Verification items for the finished model (mm, model axes). A direction names the side the tool comes from. Give positions to 0.01 mm unless a question says otherwise; leave off trailing zeros. Write each loop counter-clockwise with the first axis right and the second up, starting at its lowest first coordinate (ties: lowest second). Pieces come first, ordered by that corner, then holes. Notation, with made-up numbers: (-17, 13) -> (37, 13) arc R24 ccw to (37, 50) -> close; hole circle Ø1 at (20, 13.25). An arc over 180 degrees is marked (long way). Answer as CSV lines item,"result". Start each with the question number.
1) Sectioned sample at D-D on z = 0. Record the cut outline in (x, y).
2) Material ranges on L1, parallel to X at y = 4.25, z = -4.5; L2, parallel to Y at x = 0.5, z = -6.25; L3, parallel to X at y = 8.5, z = 0, recorded low to high.
3) Sectioned sample at B-B on z = -7. Record the cut outline in (x, y).
4) Sectioned sample at C-C on y = 11.5. Record the cut outline in (x, z).
5) Sectioned sample at A-A on x = 6. Record the cut outline in (y, z).
6) Tool access check on faces 1 (the flat face through (10, 6, 6)), 2 (the cylindrical face through (13.468, 14.409, 0.759)), 3 (the flat face through (-7, 8, -3)), 4 (the flat face through (4, 6, 0)), 5 (the flat face through (10, 6, -6)). Record the directions out of +Z, -Z, +X, -X, +Y, -Y that give a thin tool (end or side, any length) a straight path to the whole face; none if there is none.
7) Mould release check, pull along X, two halves, no side actions. Record for faces 6 (the flat face through (-11, 8, -6)), 7 (the flat face through (-3.5, 8, -6)), 8 (the flat face through (16, 4, 0)), 9 (the flat face through (0, 0, 0)): released by +X, released by -X, zero draft, split by the parting line, or undercut.
8) Gauge pin test, flat ends, axial feed: pin 1 Ø4 at (x, z) = (11, 4.5) entering from +Y; pin 2 Ø10 at (y, z) = (12.5, -5) entering from -X; pin 3 Ø6 at (x, y) = (-8, 9.5) entering from +Z; pin 4 Ø6.5 at (x, z) = (-8.5, -5.5) entering from +Y. Record the tip position at first contact, or that the pin passes through.
```python
from build123d import *

# Parameters (mm, degrees)
SKETCH1_W           = 32
SKETCH1_H           = 18
PCB_DEPTH           = 4
SKETCH2_W           = 7.5
SKETCH2_H           = 6
CONNECTOR_DEPTH     = 8
SKETCH3_W           = 12
SKETCH3_H           = 12
ENCODER_DEPTH       = 4
SKETCH4_R           = 3.5
BOSS_EXTRUDE4_DEPTH = 13


with BuildPart() as part:
    # Sketch1 → PCB (new body)
    with BuildSketch(Plane(origin=(0, 0, 0), x_dir=(1, 0, 0), z_dir=(0, 1, 0))):
        Rectangle(SKETCH1_W, SKETCH1_H)
    extrude(amount=PCB_DEPTH)

    # Sketch2 → Connector (add)
    with BuildSketch(Plane(origin=(0, 4, 0), x_dir=(1, 0, 0), z_dir=(0, 1, 0))):
        with Locations((-7.25, 6)):
            Rectangle(SKETCH2_W, SKETCH2_H)
    extrude(amount=CONNECTOR_DEPTH)

    # Sketch3 → Encoder (add)
    with BuildSketch(Plane(origin=(0, 4, 0), x_dir=(1, 0, 0), z_dir=(0, 1, 0))):
        with Locations((10, 0)):
            Rectangle(SKETCH3_W, SKETCH3_H)
    extrude(amount=ENCODER_DEPTH)

    # Sketch4 → Boss-Extrude4 (add)
    with BuildSketch(Plane(origin=(0, 8, 0), x_dir=(1, 0, 0), z_dir=(0, 1, 0))):
        with Locations(Location((10.051012923, 0, 0), (0, 0, 90))):
            Circle(SKETCH4_R)
    extrude(amount=BOSS_EXTRUDE4_DEPTH)


solid = part.part
```
Ans:
1,outline,"(-16, 0) -> (16, 0) -> (16, 8) -> (13.55, 8) -> (13.55, 21) -> (6.55, 21) -> (6.55, 8) -> (4, 8) -> (4, 4) -> (-16, 4) -> close"
2,L1,"x = -11 to -3.5, 4 to 16"
2,L2,"y = 0 to 4"
2,L3,"x = 6.55 to 13.55"
3,outline,"(-16, 0) -> (16, 0) -> (16, 4) -> (-3.5, 4) -> (-3.5, 12) -> (-11, 12) -> (-11, 4) -> (-16, 4) -> close"
4,outline,"(-11, -9) -> (-3.5, -9) -> (-3.5, -3) -> (-11, -3) -> close; circle Ø7 at (10.05, 0)"
5,outline,"(0, -9) -> (4, -9) -> (4, -6) -> (8, -6) -> (8, 6) -> (4, 6) -> (4, 9) -> (0, 9) -> close"
6,face 1,"+Z, +X, -X, +Y"
6,face 2,"+Y"
6,face 3,"+Z, -X, +Y"
6,face 4,"+Z, -Z, +Y"
6,face 5,"-Z, +X, +Y"
7,face 6,"released by -X"
7,face 7,"undercut"
7,face 8,"released by +X"
7,face 9,"zero draft"
8,pin 1,"stops at y = 21"
8,pin 2,"stops at x = -11"
8,pin 3,"stops at z = -3"
8,pin 4,"stops at y = 12"
